```python
from build123d import *

# Parameters (mm, degrees)
F0_W     = 4
F0_H     = 3.175
F0_W_2   = 3.175
F0_H_2   = 4
F1_DEPTH = 3.175


# Not quite as in the source:
# - a length typed as a fraction of an inch, garbled in the dataset ("3 / 203.2 mm" for 3/8 in), is restored


with BuildPart() as f1:
    # F0 (on Top) → F1 (new body)
    with BuildSketch(Plane.XY):
        Polygon((-25.6521557152, 6.6896411628), (-25.6521557152, 8.1896411628), (-22.6521557152, 8.1896411628), (-22.6521557152, 6.6896411628), (-21.1521557152, 6.6896411628), (-21.1521557152, 4.6896411628), (-22.6521557152, 4.6896411628), (-22.6521557152, 1.3646411628), (-19.6521557152, 1.3646411628), (-15.6521557152, 1.3646411628), (-13.6521557152, 1.3646411628), (-13.6521557152, 5.3646411628), (-13.6521557152, 8.3646411628), (-16.9771557152, 8.3646411628), (-16.9771557152, 6.8646411628), (-18.9771557152, 6.8646411628), (-18.9771557152, 8.3646411628), (-20.4771557152, 8.3646411628), (-20.4771557152, 11.3646411628), (-18.9771557152, 11.3646411628), (-18.9771557152, 12.8646411628), (-16.9771557152, 12.8646411628), (-16.9771557152, 11.3646411628), (-13.6521557152, 11.3646411628), (-13.6521557152, 14.3646411628), (-13.6521557152, 18.3646411628), (-19.7197964023, 18.3646411628), (-32.6521557152, 5.4322818499), (-32.6521557152, 1.3646411628), (-28.6521557152, 1.3646411628), (-25.6521557152, 1.3646411628), (-25.6521557152, 4.6896411628), (-27.1521557152, 4.6896411628), (-27.1521557152, 6.6896411628), align=None)
        with Locations((-30.6521557152, -0.2228588372)):
            Rectangle(F0_W, F0_H)
        with Locations((-17.6521557152, -0.2228588372)):
            Rectangle(F0_W, F0_H)
        with Locations((-12.0646557152, 16.3646411628)):
            Rectangle(F0_W_2, F0_H_2)
    extrude(amount=F1_DEPTH)


solid = f1.part
```
Read the model definition and answer for the solid it produces. Units are mm, in the model's axes. A direction names the side the tool comes from. Give positions to 0.01 mm unless a question says otherwise; leave off trailing zeros. Order: outer loops, then holes, each group sorted by start corner. A loop starts at its lowest first (then second) coordinate and runs counter-clockwise, first axis right, second up.
(1) For a pull along X with two mould halves and no side action, classify faces 1 (the flat face through (-15.652, 0, 2)), 2 (the flat face through (-15, 8.365, 2)), 3 (the flat face through (-19.652, 0, 2)) as released by +X, released by -X, zero draft, split by the parting line, or undercut.
(2) Straight lines are drawn through the part: L1, parallel to Y at x = -15.75, z = 3; L2, parallel to Y at x = -17.25, z = 2.1; L3, parallel to X at y = 0.75, z = 0.4. For each, find the intervals that lie inside material, in ascending order.
(3) Find section C-C (y = 16). Give the vertices of the cut face in (x, z) (3 decimals), plus the area to 3 significant figures.
(4) Find section D-D (x = -23.75). Give the vertices of the cut face in (y, z) (3 decimals).
(5) For faces 4 (the flat face through (-22, 6.69, 2)), 5 (the flat face through (-12, 14.365, 2)), 6 (the flat face through (-32.652, 2, 2)), 7 (the flat face through (-15, 11.365, 2)), 8 (the flat face through (-22.652, 3, 2)), determine the directions among +Z, -Z, +X, -X, +Y, -Y from which every point of the face is accessible in a straight line to the end or side of a thin tool.
(6) Find section A-A (y = 2.5). Give the vertices of the cut face in (x, z) (3 decimals).
(7) Given pin 1 (1.5 mm diameter, centred on x = -21.5, z = 2, fed in from -Y); pin 2 (1 mm diameter, centred on y = 0, z = 2, fed in from +X); pin 3 (1.6 mm diameter, centred on x = -22, z = 1, fed in from +Y), each flat-ended and moving along its own axis, determine where each tip first touches the part or whether it passes through.
(8) Find section B-B (x = -16). Give the vertices of the cut face in (y, z) (3 decimals), plus the area to 3 significant figures.
Result sheet:
1. face 1: released by +X
1. face 2: zero draft
1. face 3: undercut
2. L1: y = -1.81 to 8.36, 11.36 to 18.36
2. L2: y = -1.81 to 6.86, 12.86 to 18.36
2. L3: x = -32.65 to -28.65, -19.65 to -15.65
3. outline: (-22.084, 0) - (-10.477, 0) - (-10.477, 3.175) - (-22.084, 3.175) - close
3. area: 36.9 mm2
4. outline: (8.19, 0) - (14.334, 0) - (14.334, 3.175) - (8.19, 3.175) - close
5. face 4: +Z, -Z
5. face 5: +Z, -Z, +X, -Y
5. face 6: +Z, -Z, -X, +Y, -Y
5. face 7: +Z, -Z, +X
5. face 8: +Z, -Z, -Y
6. outline: (-32.652, 0) - (-25.652, 0) - (-25.652, 3.175) - (-32.652, 3.175) - close; (-22.652, 0) - (-13.652, 0) - (-13.652, 3.175) - (-22.652, 3.175) - close
7. pin 1: stops at y = 1.36
7. pin 2: stops at x = -15.65
7. pin 3: stops at y = 16.88
8. outline: (-1.81, 0) - (8.365, 0) - (8.365, 3.175) - (-1.81, 3.175) - close; (11.365, 0) - (18.365, 0) - (18.365, 3.175) - (11.365, 3.175) - close
8. area: 54.5 mm2
